Geometry: final body of the model. Coordinates: model frame, mm. Give positions to 0.01 mm unless a question says otherwise; leave off trailing zeros. Order: outer loops, then holes, each group sorted by start corner. A loop starts at its lowest first (then second) coordinate and runs counter-clockwise, first axis right, second up. Notation, with made-up numbers: (-35, -15) - (-7, -15) arc R11 cw to (-7, 5) - close; hole circle Ø8 at (-0.5, -20.5). An arc over 180 degrees is marked (long way). Write item = value, one per line. Start each with the question number.
from build123d import *

# Parameters (mm, degrees)
SKETCH_1_R          = 1
SKETCH_1_R_2        = 3
EXTRUDE_1_DEPTH     = 2
CUT_EXTRUDE_START   = -10
CUT_EXTRUDE_1_DEPTH = 10
FILLET_1_R          = 2
CHAMFER_1_SIZE      = 0.866


with BuildPart() as part:
    # 草图1 → 凸台-拉伸1 (new body)
    with BuildSketch(Plane.XY):
        with BuildLine():
            Line((-9.604686356, 8), (9.604686356, 8))
            ThreePointArc((9.604686356, 8), (0, -12.5), (-9.604686356, 8))
        make_face()
        with Locations((0, -10.5)):
            Circle(SKETCH_1_R, mode=Mode.SUBTRACT)
        with Locations((-9.09326674, 5.25)):
            Circle(SKETCH_1_R, mode=Mode.SUBTRACT)
        with Locations((9.09326674, 5.25)):
            Circle(SKETCH_1_R, mode=Mode.SUBTRACT)
        with Locations((-5.75, 0)):
            Circle(SKETCH_1_R, mode=Mode.SUBTRACT)
        with Locations(Location((5.75, 0, 0), (0, 0, 180))):
            Circle(SKETCH_1_R, mode=Mode.SUBTRACT)
        Circle(SKETCH_1_R_2, mode=Mode.SUBTRACT)
    extrude(amount=EXTRUDE_1_DEPTH)

    # 草图2 → 切除-拉伸1 (cut)
    with BuildSketch(Plane.XY.offset(2).offset(CUT_EXTRUDE_START)):
        with BuildLine():
            ThreePointArc((-11.98818711, -3.540249967), (-6.363961031, -6.363961031), (-3.540249967, -11.98818711))
            ThreePointArc((-3.540249967, -11.98818711), (-8.838834765, -8.838834765), (-11.98818711, -3.540249967))
        make_face()
        with BuildLine():
            ThreePointArc((11.98818711, -3.540249967), (6.363961031, -6.363961031), (3.540249967, -11.98818711))
            ThreePointArc((3.540249967, -11.98818711), (8.838834765, -8.838834765), (11.98818711, -3.540249967))
        make_face()
    extrude(amount=CUT_EXTRUDE_1_DEPTH, mode=Mode.SUBTRACT)

    # 圆角1
    fillet_1_edges = [part.edges().sort_by_distance(p)[0] for p in [
        (-3.540249967, -11.98818711, 1),
        (-11.98818711, -3.540249967, 1),
        (-9.604686356, 8, 1),
        (11.98818711, -3.540249967, 1),
        (9.604686356, 8, 1),
        (3.540249967, -11.98818711, 1),
    ]]
    fillet(fillet_1_edges, radius=FILLET_1_R)

    # 倒角1
    chamfer_1_edges = [part.edges().sort_by_distance(p)[0] for p in [
        (-6.75, 0, 2),
        (6.75, 0, 2),
    ]]
    chamfer(chamfer_1_edges, length=CHAMFER_1_SIZE)


solid = part.part
Q1. Section C-C, the plane y = 2.25. Return the cut outline in (x, z), then the cut area to 3 significant figures.
Q2. Material intervals for line 1 along Y through (x, z) = (0, 0.7); line 2 along X through (y, z) = (-0.25, 0.85); line 3 along Y through (x, z) = (5.75, 0.3), sorted ascending. Write a range as from..to.
Q3. Pull-direction query (X, two-part tool) for faces 1 (the cylindrical face through (8.36, 5.93, 0.99)), 2 (the cylindrical face through (-6.42, -6.31, 0.99)), 3 (the flat face through (-3, -2, 0)), 4 (the cylindrical face through (0, -12.5, 1)); classes: +X half, -X half, draft (parallel to the pull), parting line (faces both ways), or undercut.
Q4. Section D-D, the plane y = 5.25. Return the cut outline in (x, z).
Q5. Contact query for flat-ended pins moving along their axis: pin 1 (1.2 mm diameter, centred on x = 5.75, y = 0, fed in from -Z); pin 2 (1 mm diameter, centred on y = -9, z = 1, fed in from +X). Output: stop coordinate, or through.
Q6. Section B-B, the plane x = -5.75. Return the cut outline in (y, z).
Q7. Section A-A, the plane y = 0. Return the cut outline in (x, z).
The answers:
q1.outline = (-12.3, 0) - (-1.98, 0) - (-1.98, 2) - (-12.3, 2) - close; (1.98, 0) - (12.3, 0) - (12.3, 2) - (1.98, 2) - close
q1.area = 41.2 mm²
q2.line_1 = -12.5..-11.5, -9.5..-3, 3..8
q2.line_2 = -12.5..-6.72, -4.78..-2.99, 2.99..4.78, 6.72..12.5
q2.line_3 = -7.04..-1, 1..8
q3.face_1 = undercut
q3.face_2 = -X half
q3.face_3 = draft
q3.face_4 = parting line
q4.outline = (-11.34, 0) - (-10.09, 0) - (-10.09, 2) - (-11.34, 2) - close; (-8.09, 0) - (8.09, 0) - (8.09, 2) - (-8.09, 2) - close; (10.09, 0) - (11.34, 0) - (11.34, 2) - (10.09, 2) - close
q5.pin_1 = through
q5.pin_2 = 4.74
q6.outline = (-7.04, 0) - (-1, 0) - (-1, 1.13) - (-1.87, 2) - (-7.04, 2) - close; (1, 0) - (8, 0) - (8, 2) - (1.87, 2) - (1, 1.13) - close
q7.outline = (-12.5, 0) - (-6.75, 0) - (-6.75, 1.13) - (-7.62, 2) - (-12.5, 2) - close; (-4.75, 0) - (-3, 0) - (-3, 2) - (-3.88, 2) - (-4.75, 1.13) - close; (3, 0) - (4.75, 0) - (4.75, 1.13) - (3.88, 2) - (3, 2) - close; (6.75, 0) - (12.5, 0) - (12.5, 2) - (7.62, 2) - (6.75, 1.13) - close
